from build123d import *

# Parameters (mm, degrees)
SKETCH1_W           = 20
SKETCH1_H           = 10
BOSS_EXTRUDE1_DEPTH = 3
SKETCH2_R           = 1.5
BOSS_EXTRUDE2_DEPTH = 50
SKETCH3_R           = 2.5
BOSS_EXTRUDE3_DEPTH = 30


with BuildPart() as part:
    # Sketch1 → Boss-Extrude1 (new body)
    with BuildSketch(Plane(origin=(0, 0, 0), x_dir=(1, 0, 0), z_dir=(0, 1, 0))):
        Rectangle(SKETCH1_W, SKETCH1_H)
    extrude(amount=BOSS_EXTRUDE1_DEPTH)

    # Sketch2 → Boss-Extrude2 (add)
    with BuildSketch(Plane(origin=(0, 3, 0), x_dir=(1, 0, 0), z_dir=(0, 1, 0))):
        with Locations((-5, 0)):
            Circle(SKETCH2_R)
        with Locations((5, 0)):
            Circle(SKETCH2_R)
    extrude(amount=BOSS_EXTRUDE2_DEPTH)

    # Sketch3 → Boss-Extrude3 (add)
    with BuildSketch(Plane.XZ):
        Circle(SKETCH3_R)
    extrude(amount=BOSS_EXTRUDE3_DEPTH)


solid = part.part
Model file for the job. Use its own axes, mm. A direction names the side the tool comes from. Give positions to 0.01 mm unless a question says otherwise; leave off trailing zeros. Order: outer loops, then holes, each group sorted by start corner. A loop starts at its lowest first (then second) coordinate and runs counter-clockwise, first axis right, second up. Notation, with made-up numbers: M 25,59.25 L 41,59.25 A12 cw 41,71.25 Z; hole C 8.5,68 d7. An arc over 180 degrees is marked long. Put each result on its own line as item: value. Start each with the question number.
(1) Pull direction X, two halves, no side cores. Call faces 4 (the face through (-6.2, 27.6, 0.9)), 5 (the face through (-0.54, -14.79, -2.44)), 6 (the face through (0, 1, 5)), 7 (the face through (10, 1, 0)): released by +X, released by -X, zero draft, split by the parting line, or undercut.
(2) Drill centre lines: L1, parallel to X at y = 43, z = 0; L2, parallel to Y at x = -5.5, z = 3; L3, parallel to X at y = 5, z = -0.75. Where is each one in solid material? Low to high. Write a range as [from, to].
(3) Band-saw the part on B-B on y = 19. Give the cut face in (x, z), then the cut area to 3 significant figures.
(4) Tool access for faces 1 (the face through (6.386, 27.65, 0.575)), 2 (the face through (5, 53, 0)), 3 (the face through (-2.4, 0, -1.2)): list every direction of +Z, -Z, +X, -X, +Y, -Y with a clear straight run to the whole face (end or side of a thin tool).
(5) Band-saw the part on A-A on z = 0. Give the cut face in (x, y).
(6) Band-saw the part on C-C on x = -5. Give the cut face in (y, z).
(7) Pin check, flat tips, straight feed: pin 1 Ø2 at (x, y) = (-3, -1.5) entering from -Z; pin 2 Ø3 at (x, y) = (-1.5, -5) entering from +Z; pin 3 Ø10 at (x, y) = (-6, -18) entering from -Z; pin 4 Ø5 at (x, y) = (-6, -5.5) entering from -Z. Stop position of each tip, or through.
(8) Band-saw the part on D-D on y = -2.5. Give the cut face in (x, z), then the cut area to 3 significant figures.
Results below:
1. face 4: undercut
1. face 5: split by the parting line
1. face 6: zero draft
1. face 7: released by +X
2. L1: x = [-6.5, -3.5], [3.5, 6.5]
2. L2: y = [0, 3]
2. L3: x = [-6.3, -3.7], [3.7, 6.3]
3. outline: C -5,0 d3; C 5,0 d3
3. area: 14.1 mm2
4. face 1: +Y
4. face 2: +Z, -Z, +X, -X, +Y
4. face 3: -Y
5. outline: M -10,0 L -2.5,0 L -2.5,-30 L 2.5,-30 L 2.5,0 L 10,0 L 10,3 L 6.5,3 L 6.5,53 L 3.5,53 L 3.5,3 L -3.5,3 L -3.5,53 L -6.5,53 L -6.5,3 L -10,3 Z
6. outline: M 0,-5 L 3,-5 L 3,-1.5 L 53,-1.5 L 53,1.5 L 3,1.5 L 3,5 L 0,5 Z
7. pin 1: stops at z = -1.5
7. pin 2: stops at z = 2.5
7. pin 3: stops at z = -2.29
7. pin 4: passes through
8. outline: C 0,0 d5
8. area: 19.6 mm2
